```python
from build123d import *

# Parameters (mm, degrees)
SKETCH_1_W          = 17.893001423
SKETCH_1_H          = 11.620982588
SKETCH_1_H_2        = 11.620982589
EXTRUDE_1_DEPTH     = 2
SKETCH_2_R          = 1.5
CUT_EXTRUDE_1_DEPTH = 10
CHAMFER_1_SIZE      = 1
SKETCH_3_R          = 1.5
CUT_EXTRUDE_2_DEPTH = 10
SKETCH_4_W          = 33.95700602
SKETCH_4_H          = 96
CUT_EXTRUDE_3_DEPTH = 10
CHAMFER_2_SIZE      = 1


with BuildPart() as part:
    # Эскиз1 → Бобышка-Вытянуть1 (new body)
    with BuildSketch(Plane(origin=(0, 0, 0), x_dir=(1, 0, 0), z_dir=(0, 1, 0))):
        Polygon((49.933797981, 26), (18.309932441, 26), (18.309932441, 48), (15, 48), (-48.959081244, 48), (-48.959081244, -48), (15, -48), (18.309932441, -48), (18.309932441, -26), (49.933797981, -26), align=None)
        with Locations((-36.319088007, -31.12001489)):
            Rectangle(SKETCH_1_W, SKETCH_1_H, mode=Mode.SUBTRACT)
        with Locations((-36.319088007, 31.12001489)):
            Rectangle(SKETCH_1_W, SKETCH_1_H_2, mode=Mode.SUBTRACT)
    extrude(amount=EXTRUDE_1_DEPTH)

    # Эскиз2 → Вырез-Вытянуть1 (cut)
    with BuildSketch(Plane(origin=(0, 2, 0), x_dir=(1, 0, 0), z_dir=(0, 1, 0))):
        with Locations(Location((46.183797981, -14.4, 0), (0, 0, 270))):
            Circle(SKETCH_2_R)
        with Locations(Location((18.683797981, -14.4, 0), (0, 0, 270))):
            Circle(SKETCH_2_R)
        with Locations(Location((18.683797981, -4.4, 0), (0, 0, 270))):
            Circle(SKETCH_2_R)
        with Locations(Location((46.183797981, -4.4, 0), (0, 0, 270))):
            Circle(SKETCH_2_R)
        with Locations(Location((18.683797981, 5.6, 0), (0, 0, 270))):
            Circle(SKETCH_2_R)
        with Locations(Location((46.183797981, 5.6, 0), (0, 0, 270))):
            Circle(SKETCH_2_R)
        with Locations(Location((18.683797981, 15.6, 0), (0, 0, 270))):
            Circle(SKETCH_2_R)
        with Locations(Location((46.183797981, 15.6, 0), (0, 0, 270))):
            Circle(SKETCH_2_R)
    extrude(amount=-CUT_EXTRUDE_1_DEPTH, mode=Mode.SUBTRACT)

    # Фаска1
    chamfer_1_edges = [part.edges().sort_by_distance(p)[0] for p in [
        (46.183797981, 0, -7.1),
        (18.683797981, 0, 2.9),
        (46.183797981, 0, 2.9),
        (18.683797981, 0, 12.9),
        (18.683797981, 0, -17.1),
        (46.183797981, 0, -17.1),
        (18.683797981, 0, -7.1),
        (46.183797981, 0, 12.9),
    ]]
    chamfer(chamfer_1_edges, length=CHAMFER_1_SIZE)

    # Эскиз3 → Вырез-Вытянуть2 (cut)
    with BuildSketch(Plane(origin=(0, 2, 0), x_dir=(1, 0, 0), z_dir=(0, 1, 0))):
        with Locations(Location((5.923569009, 32.746976788, 0), (0, 0, 270))):
            Circle(SKETCH_3_R)
        with Locations(Location((-2.726430991, 32.746976788, 0), (0, 0, 270))):
            Circle(SKETCH_3_R)
        with Locations(Location((-2.726430991, -35.660220789, 0), (0, 0, 270))):
            Circle(SKETCH_3_R)
        with Locations(Location((5.923569009, -35.660220789, 0), (0, 0, 270))):
            Circle(SKETCH_3_R)
    extrude(amount=-CUT_EXTRUDE_2_DEPTH, mode=Mode.SUBTRACT)

    # Эскиз4 → Вырез-Вытянуть3 (cut)
    with BuildSketch(Plane(origin=(0, 2, 0), x_dir=(1, 0, 0), z_dir=(0, 1, 0))):
        with Locations((-31.980578234, 0)):
            Rectangle(SKETCH_4_W, SKETCH_4_H)
    extrude(amount=-CUT_EXTRUDE_3_DEPTH, mode=Mode.SUBTRACT)

    # Фаска2
    chamfer_2_edges = [part.edges().sort_by_distance(p)[0] for p in [
        (5.923569009, 0, 34.160220789),
        (-2.726430991, 0, 34.160220789),
        (-2.726430991, 0, -34.246976788),
        (5.923569009, 0, -34.246976788),
    ]]
    chamfer(chamfer_2_edges, length=CHAMFER_2_SIZE)


solid = part.part
```
Here's how the part is built. I have some questions about the finished solid (model axes, mm). A direction names the side the tool comes from. Give positions to 0.01 mm unless a question says otherwise; leave off trailing zeros. Write each loop counter-clockwise with the first axis right and the second up, starting at its lowest first coordinate (ties: lowest second). Pieces come first, ordered by that corner, then holes. Notation, with made-up numbers: M 59,80 L 81,80 A20 cw 81,112 Z; hole C 73.5,-16.75 d5. An arc over 180 degrees is marked long. Put each result on its own line as item: value. Start each with the question number.
Item 1: On a 3-axis mill with a long thin cutter (end or side, diameter ignored), from which of +Z, -Z, +X, -X, +Y, -Y can I reach the whole of each face in a straight line? I mean faces 5 (the flat face through (34, 1, 26)), 6 (the cylindrical face through (47.198, 1.507, 13.294)), 7 (the flat face through (34, 1, -26)). Say none if no direction works.
Item 2: If we section it at B-B, the plane y = 0.55: Count the separate pieces of the cut face and the enclosed holes in it, then the cut area to 3 significant figures.
Item 3: If we section it at C-C, the plane x = 25: Write out the boundary of the cut face in (y, z), then the cut area to 3 significant figures.
Item 4: Thinking about a two-plate mould opening in X: for faces 1 (the flat face through (-15.002, 1, 1)), 2 (the flat face through (49.934, 1, 0)), 3 (the flat face through (1, 1, 48)), 4 (the cylindrical face through (19.698, 1.507, 13.294)), which applies, +X half, -X half, draft (parallel to the pull), parting line (faces both ways), or undercut?
Item 5: If we section it at D-D, the plane z = -39: Write out the boundary of the cut face in (x, y), then the cut area to 3 significant figures.
Item 6: Will these pins go through, and if not, where does the flat tip stop? pin 1 (3.5 mm diameter, centred on x = 46.18, z = 14.4, fed in from -Y); pin 2 (1 mm diameter, centred on y = 0.5, z = -34.5, fed in from +X); pin 3 (0.6 mm diameter, centred on x = 40, y = 0.5, fed in from -Z).
Item 7: If we section it at A-A, the plane z = 14.4: Write out the boundary of the cut face in (x, y), then the cut area to 3 significant figures.
Item 8: I need wall thicknesses on L1, parallel to X at y = 1.2, z = 4.4; L2, parallel to X at y = 1.1, z = -33; L3, parallel to Z at x = -2.5, y = 1.3. Which ranges of each line are inside material? Lowest first, please. Write a range as from..to.
Values:
1. face 5: +Z, +X, +Y, -Y
1. face 6: +Y, -Y
1. face 7: -Z, +X, +Y, -Y
2. separate pieces: 1
2. enclosed holes: 12
2. area: 4,700 mm²
3. outline: M 0,-26 L 2,-26 L 2,26 L 0,26 Z
3. area: 104 mm²
4. face 1: -X half
4. face 2: +X half
4. face 3: draft
4. face 4: undercut
5. outline: M -15,0 L 18.31,0 L 18.31,2 L -15,2 Z
5. area: 66.6 mm²
6. pin 1: y = 0.75
6. pin 2: x = 18.31
6. pin 3: z = -26
7. outline: M -15,0 L 16.18,0 L 17.18,1 L 17.18,2 L -15,2 Z; M 20.18,1 L 21.18,0 L 43.68,0 L 44.68,1 L 44.68,2 L 20.18,2 Z; M 47.68,1 L 48.68,0 L 49.93,0 L 49.93,2 L 47.68,2 Z
7. area: 116 mm²
8. L1: -15..17.18, 20.18..44.68, 47.68..49.93
8. L2: -15..-4.2, -1.25..4.45, 7.4..18.31
8. L3: -48..-34.23, -31.26..34.18, 37.14..48
